from build123d import *

# Parameters (mm, degrees)
BOSS_EXTRUDE1_DEPTH = 7.5
SKETCH2_R           = 3
CUT_EXTRUDE1_DEPTH  = 15


with BuildPart() as part:
    # Sketch1 → Boss-Extrude1 (new, symmetric)
    with BuildSketch(Plane(origin=(0, 0, 0), x_dir=(-1, 0, 0), z_dir=(0, 0, 1))):
        with BuildLine():
            Line((5.154406377, -5.123005585), (3.963575151, 3.922255592))
            ThreePointArc((3.963575151, 3.922255592), (0, 3.846483961), (-3.963575151, 3.922255592))
            Line((-3.963575151, 3.922255592), (-5.154406377, -5.123005585))
            ThreePointArc((-5.154406377, -5.123005585), (0, -5.241098686), (5.154406377, -5.123005585))
        make_face()
    extrude(amount=BOSS_EXTRUDE1_DEPTH, both=True)

    # Sketch2 → Cut-Extrude1 (cut)
    with BuildSketch(Plane.XY.offset(7.5)):
        with Locations((0, 0.600374996)):
            Circle(SKETCH2_R)
    extrude(amount=-CUT_EXTRUDE1_DEPTH, mode=Mode.SUBTRACT)


solid = part.part
Can you work these out from the model? Positions are in its coordinate system, mm. Give positions to 0.01 mm unless a question says otherwise; leave off trailing zeros. Order: outer loops, then holes, each group sorted by start corner. A loop starts at its lowest first (then second) coordinate and runs counter-clockwise, first axis right, second up. Notation, with made-up numbers: M 42.25,-5 L 59.25,-5 A19 cw 59.25,32 Z; hole C -13.5,56 d11. An arc over 180 degrees is marked long. One line per item, written item: value.
Item 1: If we section it at C-C on z = 5: Write out the boundary of the cut face in (x, y), and give its area (3 significant figures).
Verdict:
outline: M -5.15,5.12 L -3.96,-3.92 A103.7 cw 3.96,-3.92 L 5.15,5.12 A112.55 ccw Z; hole C 0,0.6 d6
area: 54.6 mm2
Item 2: Please list where these lines run through material, in increasing order: line 1 (Y direction, x = 0, z = -3.25); line 2 (X direction, y = -2, z = 6); line 3 (X direction, y = -1.5, z = -5).
Verdict:
line 1: -3.85 to -2.4, 3.6 to 5.24
line 2: -4.22 to -1.5, 1.5 to 4.22
line 3: -4.28 to -2.14, 2.14 to 4.28
Item 3: If we mould it in two halves opening along X, with no side actions, what happens to faces 1 (the face through (4.55, 0.54, 0.11)), 2 (the face through (0, 4, 7.5)), 3 (the face through (-0.056, -3.846, 0.105))? For each: pulls with the +X half, pulls with the -X half, needs draft (parallel to the pull), parting line crosses it, or undercut.
Verdict:
face 1: pulls with the +X half
face 2: needs draft
face 3: undercut
Item 4: If we section it at B-B on y = -2: Write out the boundary of the cut face in (x, z).
Verdict:
outline: M -4.22,-7.5 L -1.5,-7.5 L -1.5,7.5 L -4.22,7.5 Z; M 1.5,-7.5 L 4.22,-7.5 L 4.22,7.5 L 1.5,7.5 Z
Item 5: If we section it at A-A on x = 0: Write out the boundary of the cut face in (y, z), and give its area (3 significant figures).
Verdict:
outline: M -3.85,-7.5 L -2.4,-7.5 L -2.4,7.5 L -3.85,7.5 Z; M 3.6,-7.5 L 5.24,-7.5 L 5.24,7.5 L 3.6,7.5 Z
area: 46.3 mm2
Item 6: For pin 1 (1 mm diameter, centred on y = -1.5, z = -5.5, fed in from +X); pin 2 (2 mm diameter, centred on y = 1.5, z = 1.5, fed in from -X); pin 3 (3.5 mm diameter, centred on x = 0, y = 0.6, fed in from +Z); pin 4 (2 mm diameter, centred on y = 0.5, z = -2.5, fed in from +X), each with a flat end and sliding along its axis, tell me the tip position at first contact or that it passes through.
Verdict:
pin 1: x = 4.35
pin 2: x = -4.81
pin 3: through
pin 4: x = 4.68
Item 7: If we section it at D-D on x = 4.75: Write out the boundary of the cut face in (y, z).
Verdict:
outline: M 2.05,-7.5 L 5.14,-7.5 L 5.14,7.5 L 2.05,7.5 Z
